```python
from build123d import *

# Parameters (mm, degrees)
SKETCH1_R             = 20
BOSS_EXTRUDE1_DEPTH   = 10
SKETCH2_W             = 10
SKETCH2_H             = 10
CUT_EXTRUDE1_DEPTH    = 5
M4X0_7_TAPPED_HOLE1_D = 3.3
SKETCH6_R             = 20
SKETCH6_R_2           = 12.5
CUT_EXTRUDE2_DEPTH    = 5
M4X0_7_TAPPED_HOLE2_D = 3.3


with BuildPart() as part:
    # Sketch1 → Boss-Extrude1 (new body)
    with BuildSketch(Plane.XY):
        Circle(SKETCH1_R)
    extrude(amount=BOSS_EXTRUDE1_DEPTH)

    # Sketch2 → Cut-Extrude1 (cut)
    with BuildSketch(Plane(origin=(0, 0, 0), x_dir=(-1, 0, 0), z_dir=(0, 0, -1))):
        Rectangle(SKETCH2_W, SKETCH2_H)
    extrude(amount=-CUT_EXTRUDE1_DEPTH, mode=Mode.SUBTRACT)

    # M4x0.7 Tapped Hole1 (through all)
    with Locations(Plane.XY.offset(10)):
        with Locations((0, 0)):
            Hole(M4X0_7_TAPPED_HOLE1_D / 2)

    # Sketch6 → Cut-Extrude2 (cut)
    with BuildSketch(Plane(origin=(0, 0, 0), x_dir=(-1, 0, 0), z_dir=(0, 0, -1))):
        Circle(SKETCH6_R)
        Circle(SKETCH6_R_2, mode=Mode.SUBTRACT)
    extrude(amount=-CUT_EXTRUDE2_DEPTH, mode=Mode.SUBTRACT)

    # M4x0.7 Tapped Hole2 (through all)
    with Locations(Plane(origin=(0, 0, 5), x_dir=(-1, 0, 0), z_dir=(0, 0, -1))):
        with Locations((0, 16.5), (16.5, 0), (0, -16.5), (0, 0), (-16.5, 0)):
            Hole(M4X0_7_TAPPED_HOLE2_D / 2)


solid = part.part
```
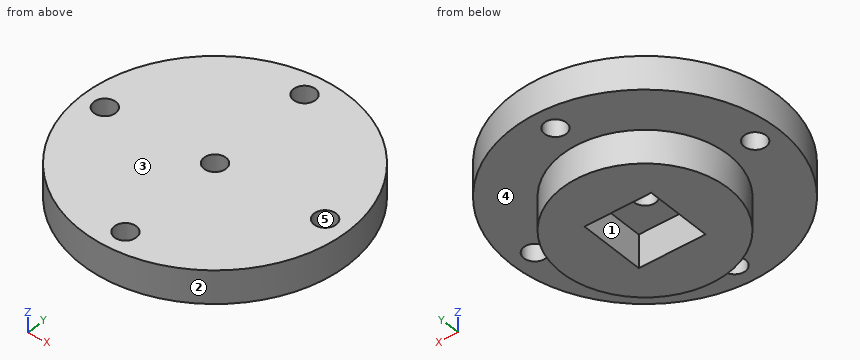
Check sheet for the modelled part. Datum: model origin and axes. Units: mm. Face numbers are marked on the shaded views. A direction names the side the tool comes from. Give positions to 0.01 mm unless a question says otherwise; leave off trailing zeros. Order: outer loops, then holes, each group sorted by start corner. A loop starts at its lowest first (then second) coordinate and runs counter-clockwise, first axis right, second up. Notation, with made-up numbers: (58.25, 7.5) -> (101.25, 7.5) arc R24 ccw to (101.25, 20.5) -> close; hole circle Ø11 at (51.25, -23.75). An arc over 180 degrees is marked (long way). Use CSV: the item, a comma, the result in double quotes. Start each with the question number.
1) Sectioned sample at D-D, the plane z = 2. Record the boundary of the cut face in (x, y).
2) Set-up check for the marked faces 4 and 5: record each of +Z, -Z, +X, -X, +Y, -Y from which the full face is reachable in a straight line by a thin tool's end or side.
3) Go/stop test with flat-tipped pins: P1, Ø1.5, axis at y = -2.5, z = 2.5, coming from the -X side; P2, Ø1, axis at x = -4.5, z = 6.5, coming from the +Y side; P3, Ø5.5, axis at x = 0, y = 0, coming from the +Z side; P4, Ø1.5, axis at x = -0.5, z = 1.5, coming from the -Y side. Record where each tip stops, or that it passes through.
4) Mould release check, pull along Y, two halves, no side actions. Record for the marked faces 1, 2 and 3: released by +Y, released by -Y, zero draft, split by the parting line, or undercut.
5) Sectioned sample at A-A, the plane x = 0. Record the boundary of the cut face in (y, z), plus the area to 4 significant figures.
6) Material ranges on line 1 (Y direction, x = 0, z = 7.6); line 2 (Z direction, x = 4, y = -17.5); line 3 (Y direction, x = 16.5, z = 7.25), recorded low to high. Write a range as from..to.
7) Sectioned sample at C-C, the plane z = 8. Record the boundary of the cut face in (x, y).
Recorded:
1,outline,"circle Ø25 at (0, 0); hole (-5, -5) -> (5, -5) -> (5, 5) -> (-5, 5) -> close"
2,face 4,"-Z"
2,face 5,"+Z, -Z"
3,P1,"x = -12.38"
3,P2,"y = 19.6"
3,P3,"z = 10"
3,P4,"y = -12.5"
4,face 1,"undercut"
4,face 2,"split by the parting line"
4,face 3,"zero draft"
5,outline,"(-20, 5) -> (-18.15, 5) -> (-18.15, 10) -> (-20, 10) -> close; (-14.85, 5) -> (-12.5, 5) -> (-12.5, 0) -> (-5, 0) -> (-5, 5) -> (-1.65, 5) -> (-1.65, 10) -> (-14.85, 10) -> close; (1.65, 5) -> (5, 5) -> (5, 0) -> (12.5, 0) -> (12.5, 5) -> (14.85, 5) -> (14.85, 10) -> (1.65, 10) -> close; (18.15, 5) -> (20, 5) -> (20, 10) -> (18.15, 10) -> close"
5,area,"225.5 mm2"
6,line 1,"-20..-18.15, -14.85..-1.65, 1.65..14.85, 18.15..20"
6,line 2,"5..10"
6,line 3,"-11.3..-1.65, 1.65..11.3"
7,outline,"circle Ø40 at (0, 0); hole circle Ø3.3 at (-16.5, 0); hole circle Ø3.3 at (0, -16.5); hole circle Ø3.3 at (0, 0); hole circle Ø3.3 at (0, 16.5); hole circle Ø3.3 at (16.5, 0)"
